Can you work these out from the model? Positions are in its coordinate system, mm. Give positions to 0.01 mm unless a question says otherwise; leave off trailing zeros. Order: outer loops, then holes, each group sorted by start corner. A loop starts at its lowest first (then second) coordinate and runs counter-clockwise, first axis right, second up.
Item 1: I'm going to push flat-ended pins straight in: pin 1 Ø5 at (x, y) = (-1160.5, 5) entering from +Z; pin 2 Ø8 at (y, z) = (5.5, -338.5) entering from +X. Where does each tip first touch, or does it pass through?
Item 2: If I drill on line 1 along X through (y, z) = (4.25, -295); line 2 along Z through (x, y) = (700, 7.25); line 3 along X through (y, z) = (6.25, 49), over which ranges is the centre line in solid material (lowest first)?
Item 3: I want a section at A-A, the plane x = 700. Write out the boundary of the cut face in (y, z).
Item 4: I want a section at B-B, the plane y = 4.75. Count the separate pieces of the cut face and the enclosed holes in it, then the cut area to 3 significant figures.
Item 5: I want a section at C-C, the plane x = -332. Write out the boundary of the cut face in (y, z).
```python
from build123d import *

# Parameters (mm, degrees)
SKETCH1_W           = 2400
SKETCH1_H           = 750
SKETCH1_R           = 30
SKETCH1_W_2         = 160
SKETCH1_H_2         = 57
BOSS_EXTRUDE1_DEPTH = 15
CUT_EXTRUDE1_START  = -75
SKETCH3_W           = 20
SKETCH3_H           = 10
CUT_EXTRUDE1_DEPTH  = 676
CUT_EXTRUDE2_START  = -675
SKETCH4_W           = 20
SKETCH4_H           = 10
CUT_EXTRUDE2_DEPTH  = 600
CUT_EXTRUDE3_START  = -2400
SKETCH4_4_W         = 20
SKETCH4_4_H         = 10
CUT_EXTRUDE3_DEPTH  = 1650
CUT_EXTRUDE4_START  = -2000
SKETCH4_5_W         = 20
SKETCH4_5_H         = 10
CUT_EXTRUDE4_DEPTH  = 1250


with BuildPart() as part:
    # Sketch1 → Boss-Extrude1 (new body)
    with BuildSketch(Plane(origin=(0, 0, 0), x_dir=(1, 0, 0), z_dir=(0, 1, 0))):
        Rectangle(SKETCH1_W, SKETCH1_H)
        with Locations((700, 295)):
            Circle(SKETCH1_R, mode=Mode.SUBTRACT)
        with Locations((420, 295)):
            Rectangle(SKETCH1_W_2, SKETCH1_H_2, mode=Mode.SUBTRACT)
    extrude(amount=BOSS_EXTRUDE1_DEPTH)

    # Sketch3 → Cut-Extrude1 (cut, through all)
    with BuildSketch(Plane(origin=(0, 0, -375), x_dir=(-1, 0, 0), z_dir=(0, 0, -1)).offset(CUT_EXTRUDE1_START)):
        with Locations((1162.5, 5)):
            Rectangle(SKETCH3_W, SKETCH3_H)
        with Locations((487.5, 5)):
            Rectangle(SKETCH3_W, SKETCH3_H)
    extrude(amount=-CUT_EXTRUDE1_DEPTH, mode=Mode.SUBTRACT)

    # Sketch4 → Cut-Extrude2 (cut)
    with BuildSketch(Plane.ZY.offset(1200).offset(CUT_EXTRUDE2_START)):
        with Locations((-337.5, 5)):
            Rectangle(SKETCH4_W, SKETCH4_H)
    extrude(amount=CUT_EXTRUDE2_DEPTH, mode=Mode.SUBTRACT)

    # Sketch4<4> → Cut-Extrude3 (cut)
    with BuildSketch(Plane.ZY.offset(1200).offset(CUT_EXTRUDE3_START)):
        with Locations((-337.5, 5)):
            Rectangle(SKETCH4_4_W, SKETCH4_4_H)
    extrude(amount=CUT_EXTRUDE3_DEPTH, mode=Mode.SUBTRACT)

    # Sketch4<5> → Cut-Extrude4 (cut)
    with BuildSketch(Plane.ZY.offset(1200).offset(CUT_EXTRUDE4_START)):
        with Locations((337.5, 5)):
            Rectangle(SKETCH4_5_W, SKETCH4_5_H)
    extrude(amount=CUT_EXTRUDE4_DEPTH, mode=Mode.SUBTRACT)


solid = part.part
```
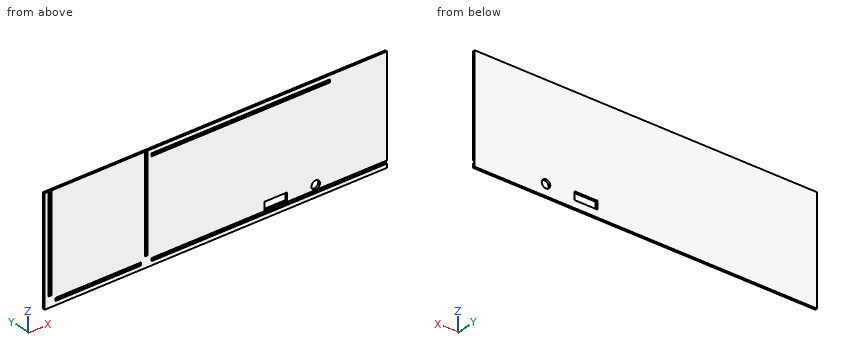
Results list:
1. pin 1: stops at z = -300
1. pin 2: stops at x = -450
2. line 1: x = -1200 to -1172.5, -1152.5 to -497.5, -477.5 to 340, 500 to 670, 730 to 1200
2. line 2: z = -375 to -347.5, -327.5 to -325, -265 to 327.5, 347.5 to 375
2. line 3: x = -1200 to -1172.5, -1152.5 to -497.5, -477.5 to 1200
3. outline: (0, -375) - (15, -375) - (15, -325) - (0, -325) - (0, -327.5) - (10, -327.5) - (10, -347.5) - (0, -347.5) - close; (0, -265) - (15, -265) - (15, 375) - (0, 375) - (0, 347.5) - (10, 347.5) - (10, 327.5) - (0, 327.5) - close
4. separate pieces: 1
4. enclosed holes: 4
4. area: 1,690,000 mm2
5. outline: (0, -375) - (15, -375) - (15, 375) - (0, 375) - (0, 347.5) - (10, 347.5) - (10, 327.5) - (0, 327.5) - (0, -327.5) - (10, -327.5) - (10, -347.5) - (0, -347.5) - close
